Geometry check sheet. Reference: the model listing, model coordinates, mm. Face numbers are marked on the shaded views. A direction names the side the tool comes from. Give positions to 0.01 mm unless a question says otherwise; leave off trailing zeros. Order: outer loops, then holes, each group sorted by start corner. A loop starts at its lowest first (then second) coordinate and runs counter-clockwise, first axis right, second up. Notation, with made-up numbers: M 51,-2 L 93,-2 A12 cw 93,2 Z; hole C -29,-7.5 d2. An arc over 180 degrees is marked long. Answer as CSV lines item,"result". Start each with the question number.
Q1. Set-up check for the marked faces 1, 2 and 3: record each of +Z, -Z, +X, -X, +Y, -Y from which the full face is reachable in a straight line by a thin tool's end or side.
Q2. Section check C-C, the plane z = 4. Record the boundary of the cut face in (x, y), then the cut area to 3 significant figures.
Q3. Go/stop test with flat-tipped pins: pin 1 (1.5 mm diameter, centred on x = 0.5, y = 0, fed in from -Z); pin 2 (4 mm diameter, centred on x = 6.5, z = 21.5, fed in from +Y); pin 3 (4 mm diameter, centred on y = -1, z = -4, fed in from +X). Record where each tip stops, or that it passes through.
Q4. Thickness scan on line 1 (Y direction, x = 0, z = 25.2); line 2 (Y direction, x = 0, z = -10.75); line 3 (Z direction, x = -3, y = -6.5). Record the ranges inside material, lowest first.
Q5. Section check A-A, the plane x = 0. Record the boundary of the cut face in (y, z).
Q6. Mould release check, pull along X, two halves, no side actions. Record for the marked faces 4, 5, 6 and 7: +X half, -X half, draft (parallel to the pull), parting line (faces both ways), or undercut.
Q7. Section check D-D, the plane z = -9.5. Record the boundary of the cut face in (x, y) (1 decimal), then the cut area to 3 significant figures.
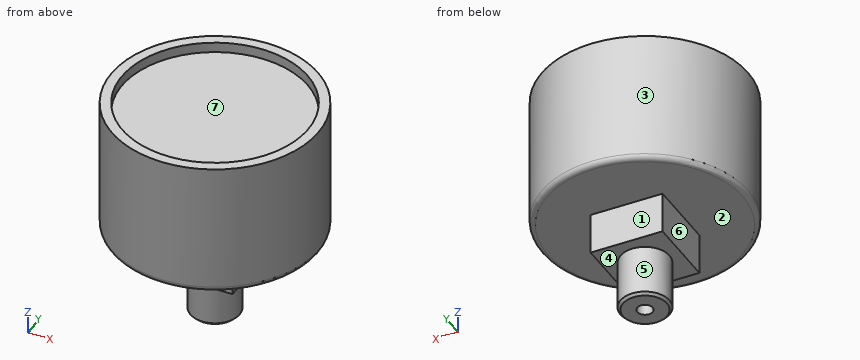
Autodesk Inventor part; units mm, degrees
ref_plane "YZ Plane" through (0, 0, 0) normal (1, 0, 0) x (0, 1, 0)
ref_plane "XZ Plane" through (0, 0, 0) normal (0, 1, 0) x (-1, 0, 0)
ref_plane "XY Plane" through (0, 0, 0) normal (0, 0, 1) x (1, 0, 0)
sketch "Sketch13" plane through (0, 0, 0) normal (0, 0, 1) x (1, 0, 0)
  circle A0 centre (0, 0) radius 20
  dimension "d46" = 40
extrude "Extrusion13" add sketch "Sketch13" along normal blind 26
sketch "Sketch15" plane through (0, 0, 0) normal (0, 0, -1) x (-1, 0, 0)
  line L0 (-7, 7) -> (7, 7)
  line L1 (7, 7) -> (7, -7)
  line L2 (7, -7) -> (-7, -7)
  line L3 (-7, -7) -> (-7, 7)
  line L4 (-28, 0) -> (28, 0)
  line L5 (0, -28) -> (0, 28)
  dimension "d52" = 14
  dimension "d53" = 14
extrude "Extrusion15" add sketch "Sketch15" along normal blind 8
sketch "Sketch16" plane through (0, 0, -8) normal (0, 0, -1) x (-1, 0, 0)
  circle A0 centre (0, 0) radius 4.7625
  dimension "d58" = 9.525
extrude "Extrusion16" add sketch "Sketch16" along normal blind 10
thread "Thread3"
sketch "Sketch18" plane through (0, 0, 26) normal (0, 0, 1) x (1, 0, 0)
  circle A0 centre (0, 0) radius 20
  circle A1 centre (0, 0) radius 18
  dimension "d66" = 2
extrude "Extrusion18" cut sketch "Sketch18" against normal blind 2 contours A1
sketch "Sketch20" plane through (0, 0, -18) normal (0, 0, -1) x (-1, 0, 0)
  circle A0 centre (0, 0) radius 4.7625
  circle A1 centre (0, 0) radius 1.5
  dimension "d75" = 3
extrude "Extrusion19" cut sketch "Sketch20" against normal blind 10 contours A1
sketch "Sketch19" plane through (0, 0, 24) normal (0, 0, 1) x (1, 0, 0)
  circle A0 centre (0, 0) radius 18
  line L0 (-6.3869, -6.5985) -> (5.7442, -6.5985) construction
  line L1 (5.7442, -6.5985) -> (5.7442, -16.6783) construction
  line L2 (5.7442, -16.6783) -> (-6.3869, -16.6783) construction
  line L3 (-6.3869, -16.6783) -> (-6.3869, -6.5985) construction
chamfer "Chamfer1" distance 0.5 angle 45 1 edges at (4.7625, 0, -18)
fillet "Fillet5" radius 1 1 edges at (-20, 0, 0)
properties part number "9690242"
Answer block:
1,face 1,"-Z, +X, -X, +Y"
1,face 2,"-Z"
1,face 3,"+Z, -Z"
2,outline,"C 0,0 d40"
2,area,"1,260 mm2"
3,pin 1,"stops at z = -8"
3,pin 2,"stops at y = 19.49"
3,pin 3,"stops at x = 7"
4,line 1,"y = -20 to -18, 18 to 20"
4,line 2,"y = -4.76 to -1.5, 1.5 to 4.76"
4,line 3,"z = -8 to 24"
5,outline,"M -20,1 A1 ccw -19,0 L -7,0 L -7,-8 L -4.76,-8 L -4.76,-17.5 L -4.26,-18 L -1.5,-18 L -1.5,-8 L 1.5,-8 L 1.5,-18 L 4.26,-18 L 4.76,-17.5 L 4.76,-8 L 7,-8 L 7,0 L 19,0 A1 ccw 20,1 L 20,26 L 18,26 L 18,24 L -18,24 L -18,26 L -20,26 Z"
6,face 4,"draft"
6,face 5,"parting line"
6,face 6,"-X half"
6,face 7,"undercut"
7,outline,"C 0,0 d9.5; hole C 0,0 d3"
7,area,"64.2 mm2"
